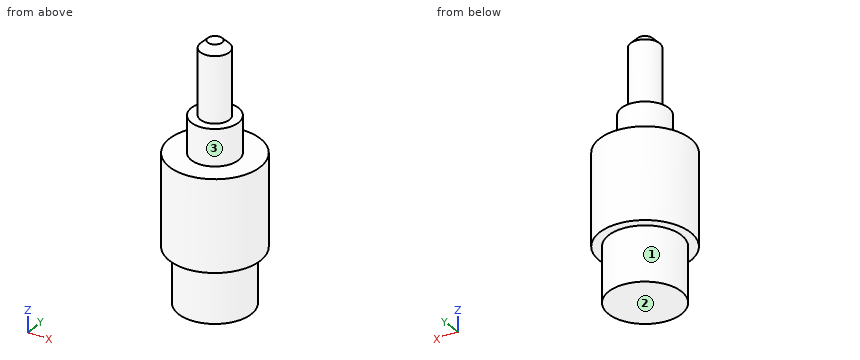
Autodesk Inventor part; units mm, degrees
ref_plane "YZ Plane" through (0, 0, 0) normal (1, 0, 0) x (0, 1, 0)
ref_plane "XZ Plane" through (0, 0, 0) normal (0, 1, 0) x (-1, 0, 0)
ref_plane "XY Plane" through (0, 0, 0) normal (0, 0, 1) x (1, 0, 0)
sketch "Sketch1" plane through (0, 0, 0) normal (0, 0, 1) x (1, 0, 0)
  circle A0 centre (0, 0) radius 12.5
  dimension "d0" = 25
extrude "Extrusion1" add sketch "Sketch1" along normal blind 25
sketch "Sketch2" plane through (0, 0, 25) normal (0, 0, 1) x (1, 0, 0)
  circle A0 centre (0, 0) radius 6.5
  dimension "d3" = 13
extrude "Extrusion2" add sketch "Sketch2" along normal blind 10
sketch "Sketch3" plane through (0, 0, 35) normal (0, 0, 1) x (1, 0, 0)
  circle A0 centre (0, 0) radius 4
  dimension "d6" = 8
extrude "Extrusion3" add sketch "Sketch3" along normal blind 20
chamfer "Chamfer1" distance 2 angle 45 1 edges at (-4, 0, 55)
sketch "Sketch4" plane through (0, 0, 0) normal (0, 0, -1) x (-1, 0, 0)
  circle A0 centre (0, 0) radius 10
  dimension "d12" = 20
extrude "Extrusion4" add sketch "Sketch4" along normal blind 15
thread "Thread1"
properties part number "dc motor"
Part model, mm, in its own coordinate system. Face numbers are marked on the shaded views. A direction names the side the tool comes from. Give positions to 0.01 mm unless a question says otherwise; leave off trailing zeros. Loops run counter-clockwise (first coordinate to the right, second up) from the corner with the lowest first, then second, coordinate; pieces in that order, holes last. Notation, with made-up numbers: M 74.5,49 L 89.5,49 A20 cw 89.5,61 Z; hole C 19.5,29.5 d7. An arc over 180 degrees is marked long. Return JSON: item names as keys, results as strings.
1) 3-axis set-ups, long thin cutter, end or side, ignore diameter. For the marked faces 1, 2 and 3: which of +Z, -Z, +X, -X, +Y, -Y reach the whole face in a straight line?
Calculated:
{"face 1": "-Z", "face 2": "-Z, +X, -X, +Y, -Y", "face 3": "+Z"}
2) Drill centre lines: line 1 (Z direction, x = 5.75, y = 1.5); line 2 (Z direction, x = 3.5, y = 8.25); line 3 (Y direction, x = -4.5, z = 31). Where is each one in solid material? Low to high.
Calculated:
{"line 1": "z = -15 to 35", "line 2": "z = -15 to 25", "line 3": "y = -4.69 to 4.69"}
3) Flat gauge pins, fed straight in: pin 1 Ø7.5 at (x, y) = (-0.5, -6) entering from +Z; pin 2 Ø3 at (y, z) = (-1.5, 31.5) entering from -X; pin 3 Ø1.5 at (y, z) = (7.5, 17.5) entering from -X; pin 4 Ø3 at (x, y) = (8, 7) entering from -Z. Where does each tip first touch, or does it go through?
Calculated:
{"pin 1": "stops at z = 54.73", "pin 2": "stops at x = -6.5", "pin 3": "stops at x = -10.52", "pin 4": "stops at z = -15"}
4) Saw through at C-C, the plane z = 40. List the corners of the cut face in (x, y).
Calculated:
{"outline": "C 0,0 d8"}
5) Saw through at D-D, the plane x = 5.25. List the corners of the cut face in (y, z), then the cut area to 3 significant figures.
Calculated:
{"outline": "M -11.34,0 L -8.51,0 L -8.51,-15 L 8.51,-15 L 8.51,0 L 11.34,0 L 11.34,25 L 3.83,25 L 3.83,35 L -3.83,35 L -3.83,25 L -11.34,25 Z", "area": "899 mm2"}
6) Saw through at A-A, the plane y = 0. List the corners of the cut face in (x, z), then the cut area to 3 significant figures.
Calculated:
{"outline": "M -12.5,0 L -10,0 L -10,-15 L 10,-15 L 10,0 L 12.5,0 L 12.5,25 L 6.5,25 L 6.5,35 L 4,35 L 4,53 L 2,55 L -2,55 L -4,53 L -4,35 L -6.5,35 L -6.5,25 L -12.5,25 Z", "area": "1,210 mm2"}
